Model file for the job. Use its own axes, mm. Face numbers are marked on the shaded views. A direction names the side the tool comes from. Round coordinates to 2 decimals unless told otherwise and drop trailing zeros. Order: outer loops, then holes, each group sorted by start corner. A loop starts at its lowest first (then second) coordinate and runs counter-clockwise, first axis right, second up. Notation, with made-up numbers: (39.25, 11.25) - (52.25, 11.25) arc R26 cw to (52.25, 27.25) - close; hole circle Ø6 at (80, -24.75). An arc over 180 degrees is marked (long way). Use one line per item in the form item = value.
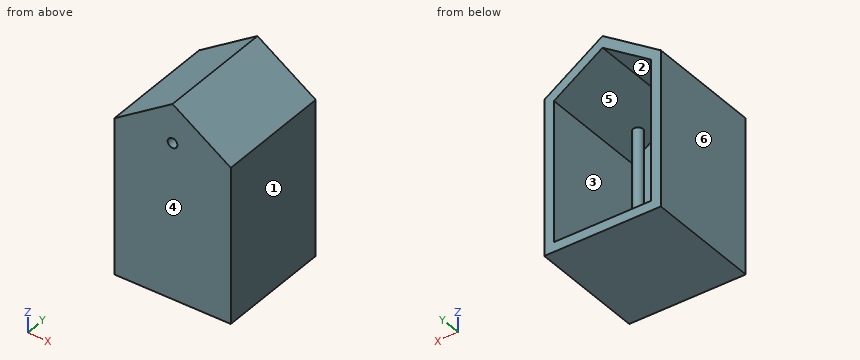
from build123d import *

# Parameters (mm, degrees)
F1_DEPTH = 38.1
F2_T     = -6.35
F5_R     = 3.2075388265
F6_DEPTH = 77.5145
F7_R     = 3.175
F8_DEPTH = 38.101


# Not quite as in the source:
# - a feature of the source that left no trace in its solid (it failed there, or was rolled back) is left out
# - the program builds the solid bodies; features that only make, move or delete a surface that nothing else refers to are left out


with BuildPart() as f1:
    # F0 (on Front) → F1 (new body, symmetric)
    with BuildSketch(Plane.XZ):
        Polygon((-38.1, 50.8), (-38.1, -50.8), (38.1, -50.8), (38.1, 50.8), (0, 76.2), align=None)
    extrude(amount=F1_DEPTH, both=True)

    # F2
    f2_openings = [f1.faces().sort_by_distance(p)[0] for p in [
        (0, 38.1, 6.585185),
    ]]
    offset(amount=F2_T, openings=f2_openings)

    # F5 (on face) → F6 (join)
    with BuildSketch(Plane.XY.offset(-44.45)):
        with Locations((0.0866505507, 6.0838097706)):
            Circle(F5_R)
    extrude(amount=F6_DEPTH)

    # F7 (on face) → F8 (cut, through all)
    with BuildSketch(Plane.XZ):
        with Locations((0, 50.8)):
            Circle(F7_R)
    extrude(amount=F8_DEPTH, mode=Mode.SUBTRACT)


solid = f1.part
(1) Slice it at A-A on y = -17. Give the cut face in (x, z).
Report:
outline = (-38.1, -50.8) - (38.1, -50.8) - (38.1, 50.8) - (0, 76.2) - (-38.1, 50.8) - close; hole (-31.75, -44.45) - (31.75, -44.45) - (31.75, 47.4) - (0, 68.57) - (-31.75, 47.4) - close
(2) Pull direction X, two halves, no side cores. Call the marked faces 3, 4, 5 and 6: released by +X, released by -X, zero draft, split by the parting line, or undercut.
Report:
face_3 = undercut
face_4 = zero draft
face_5 = undercut
face_6 = released by -X
(3) Slice it at B-B on z = 29. Give the cut face in (x, y).
Report:
outline = (-38.1, -38.1) - (38.1, -38.1) - (38.1, 38.1) - (31.75, 38.1) - (31.75, -31.75) - (-31.75, -31.75) - (-31.75, 38.1) - (-38.1, 38.1) - close; circle Ø6.42 at (0.09, 6.08)
(4) Tool access for the marked faces 1 and 2: list every direction of +Z, -Z, +X, -X, +Y, -Y with a clear straight run to the whole face (end or side of a thin tool).
Report:
face_1 = +Z, -Z, +X, +Y, -Y
face_2 = +Y
(5) Probe probe 1 along X at (y, z) = (13, 46); probe 2 along Z at (x, y) = (0, -36.75) (3 decimals); probe 3 along X at (y, z) = (-35.25, 50.8) (3 decimals). List the from-to ranges inside material, lowest first. Write a range as [from, to].
Report:
probe_1 = [-38.1, -31.75], [31.75, 38.1]
probe_2 = [-50.8, 47.625], [53.975, 76.2]
probe_3 = [-38.1, -3.175], [3.175, 38.1]
(6) Pin check, flat tips, straight feed: pin 1 (8 mm diameter, centred on x = -18, y = 17.5, fed in from +Z); pin 2 (8 mm diameter, centred on x = 16.5, y = 21, fed in from +Z); pin 3 (12 mm diameter, centred on x = 10.5, y = -29, fed in from +Z); pin 4 (8.5 mm diameter, centred on x = 0, z = 50.8, fed in from -Y). Stop position of each tip, or through.
Report:
pin_1 = 66.87
pin_2 = 67.87
pin_3 = 73.2
pin_4 = -38.1
(7) Slice it at C-C on z = 44.5. Give the cut face in (x, y).
Report:
outline = (-38.1, -38.1) - (38.1, -38.1) - (38.1, 38.1) - (31.75, 38.1) - (31.75, -31.75) - (-31.75, -31.75) - (-31.75, 38.1) - (-38.1, 38.1) - close
(8) Slice it at D-D on x = -10. Give the cut face in (y, z), then the cut area to 3 significant figures.
Report:
outline = (-38.1, -50.8) - (38.1, -50.8) - (38.1, -44.45) - (-31.75, -44.45) - (-31.75, 61.9) - (38.1, 61.9) - (38.1, 69.53) - (-38.1, 69.53) - close
area = 1,740 mm2
